```python
from build123d import *

# Parameters (mm, degrees)
CUT_EXTRUDE1_DEPTH      = 23.609258984
CUT_EXTRUDE1_DEPTH_BACK = 23.609258984
SKETCH3_W               = 2
SKETCH3_H               = 2


with BuildPart() as part:
    # Sketch1 → Revolve3 (revolve)
    with BuildSketch(Plane.XY, mode=Mode.PRIVATE) as revolve3_sk:
        Polygon((0, 0), (0, -18.924149032), (-3, -18.924149032), (-3, 0), (-6.5, 7), (-1, 7), (-1, 5), (0, 5), align=None)
    revolve(revolve3_sk.sketch.rotate(Axis((0, 5, 0), (0, -1, 0)), 270), axis=Axis((0, 5, 0), (0, -1, 0)))

    # Sketch2 → Revolve4 (revolve)
    with BuildSketch(Plane.XY, mode=Mode.PRIVATE) as revolve4_sk:
        Polygon((-3, -18.924149032), (0, -20.656199839), (0, -18.924149032), align=None)
    revolve(revolve4_sk.sketch.rotate(Axis((0, -18.924149032, 0), (0, -1, 0)), 270), axis=Axis((0, -18.924149032, 0), (0, -1, 0)))

    # Sketch3 → Cut-Extrude1 (cut, two sides: drawn at the far end of the back side and taken through both)
    with BuildSketch(Plane.XY.offset(-CUT_EXTRUDE1_DEPTH_BACK)):
        with Locations((0, 6)):
            Rectangle(SKETCH3_W, SKETCH3_H)
    extrude(amount=CUT_EXTRUDE1_DEPTH + CUT_EXTRUDE1_DEPTH_BACK, mode=Mode.SUBTRACT)


solid = part.part
```
Check sheet for the modelled part. Datum: model origin and axes. Units: mm. A direction names the side the tool comes from. Round coordinates to 2 decimals unless told otherwise and drop trailing zeros. Order: outer loops, then holes, each group sorted by start corner. A loop starts at its lowest first (then second) coordinate and runs counter-clockwise, first axis right, second up. Notation, with made-up numbers: M 31,37.5 L 89,37.5 A31 cw 89,76.5 Z; hole C 8,60 d5. An arc over 180 degrees is marked long. Answer in a Markdown table with one row per item.
(1) Material ranges on line 1 along X through (y, z) = (-4, 0); line 2 along Y through (x, z) = (2.5, -0.25); line 3 along X through (y, z) = (-8, -2), recorded low to high. Write a range as from..to.
Findings:
| item | result |
|---|---|
| line 1 | x = -3..3 |
| line 2 | y = -19.21..7 |
| line 3 | x = -2.24..2.24 |
(2) Draft check along X on faces 1 (the flat face through (1, 6, 0)), 2 (the cylindrical face through (-0.9, -9.33, 2.86)), 3 (the flat face through (-3, 7, 0)). Enter one of: +X half, -X half, draft (parallel to the pull), parting line (faces both ways), or undercut.
Findings:
| item | result |
|---|---|
| face 1 | undercut |
| face 2 | parting line |
| face 3 | draft |
(3) Gauge pin test, flat ends, axial feed: pin 1 (1.6 mm diameter, centred on y = 6.5, z = -2.5, fed in from -X); pin 2 (4 mm diameter, centred on x = -4, y = -5.5, fed in from +Z); pin 3 (5 mm diameter, centred on x = -3, y = -9, fed in from -Z). Record the tip position at first contact, or that the pin passes through.
Findings:
| item | result |
|---|---|
| pin 1 | stops at x = -6.22 |
| pin 2 | stops at z = 2.24 |
| pin 3 | stops at z = -2.96 |
(4) Set-up check for faces 4 (the conical face through (-1.2, 1.99, 3.81)), 5 (the flat face through (-1, 6, 0)): record each of +Z, -Z, +X, -X, +Y, -Y from which the full face is reachable in a straight line by a thin tool's end or side.
Findings:
| item | result |
|---|---|
| face 4 | -Y |
| face 5 | +Z, -Z, +Y |
(5) Section check A-A on y = 2. Record the boundary of the cut face in (x, z).
Findings:
| item | result |
|---|---|
| outline | C 0,0 d8 |
(6) Section check B-B on y = -11. Record the boundary of the cut face in (x, z).
Findings:
| item | result |
|---|---|
| outline | C 0,0 d6 |
